Part model, mm, in its own coordinate system. Face numbers are marked on the shaded views. A direction names the side the tool comes from. Coordinates: 2 decimals unless noted, no trailing zeros. Loops run counter-clockwise (first coordinate to the right, second up) from the corner with the lowest first, then second, coordinate; pieces in that order, holes last. Notation, with made-up numbers: M 54.25,-12 L 63.25,-12 A29 cw 63.25,12 Z; hole C 18,30.25 d10. An arc over 180 degrees is marked long. Use a Markdown table: item, result. Add a question column.
1) Tool access for the marked faces 1 and 2: list every direction of +Z, -Z, +X, -X, +Y, -Y with a clear straight run to the whole face (end or side of a thin tool).
2) Band-saw the part on C-C (y = -3). List the corners of the cut face in (x, z).
3) Band-saw the part on D-D (z = 6). List the corners of the cut face in (x, y).
4) Pull direction Z, two halves, no side cores. Call the marked faces 3, 4 and 5: released by +Z, released by -Z, zero draft, split by the parting line, or undercut.
5) Band-saw the part on A-A (x = 0). List the corners of the cut face in (y, z), plus the area to 3 significant figures.
6) Wall check: probe 1 along Y at (x, z) = (0, 4.25); probe 2 along Y at (x, z) = (0, 0.35). Give the ranges that are in metal, low to high. Write a range as from..to.
7) Pin check, flat tips, straight feed: pin 1 Ø3 at (x, y) = (0, 0) entering from +Z; pin 2 Ø1.5 at (y, z) = (2.5, 2) entering from -X; pin 3 Ø3 at (x, z) = (6, 2.5) entering from -Y; pin 4 Ø4.5 at (x, y) = (3.5, -3.5) entering from +Z. Stop position of each tip, or through.
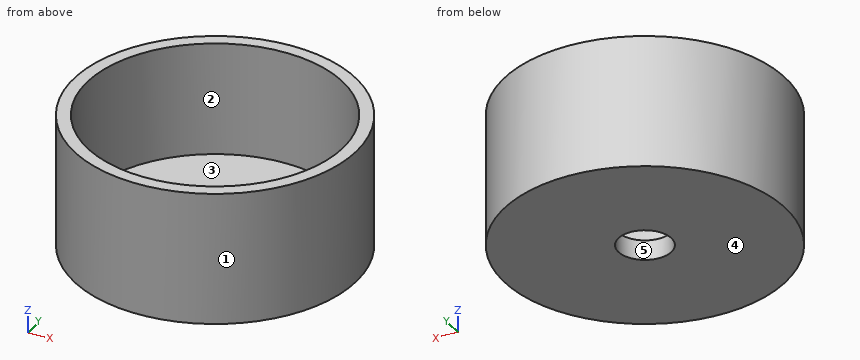
Autodesk Inventor part; units mm, degrees
ref_plane "YZ Plane" through (0, 0, 0) normal (1, 0, 0) x (0, 1, 0)
ref_plane "XZ Plane" through (0, 0, 0) normal (0, 1, 0) x (-1, 0, 0)
ref_plane "XY Plane" through (0, 0, 0) normal (0, 0, 1) x (1, 0, 0)
sketch "Sketch1" plane through (0, 0, 0) normal (0, 0, 1) x (1, 0, 0)
  circle A0 centre (0, 0) radius 8.5
  dimension "d0" = 17
extrude "Extrusion1" add sketch "Sketch1" along normal blind 8
sketch "Sketch2" plane through (0, 0, 8) normal (0, 0, 1) x (1, 0, 0)
  circle A0 centre (0, 0) radius 7.7
  circle A1 centre (0, 0) radius 8.5
  dimension "d3" = 0.8
extrude "Extrusion2" cut sketch "Sketch2" against normal blind 6.8 contours A0
sketch "Sketch3" plane through (0, 0, 0) normal (0, 0, -1) x (-1, 0, 0)
  point P0 (0, 0)
hole "Hole1" at (0, 0, 0) direction (0, 0, 1) diameter 3.2 end through all
properties part number "SpoolSpringBushing"
Entries:
| question | item | result |
|---|---|---|
| 1 | face 1 | +Z, -Z |
| 1 | face 2 | +Z |
| 2 | outline | M -7.95,0 L 7.95,0 L 7.95,8 L 7.09,8 L 7.09,1.2 L -7.09,1.2 L -7.09,8 L -7.95,8 Z |
| 3 | outline | C 0,0 d17; hole C 0,0 d15.4 |
| 4 | face 3 | released by +Z |
| 4 | face 4 | released by -Z |
| 4 | face 5 | zero draft |
| 5 | outline | M -8.5,0 L -1.6,0 L -1.6,1.2 L -7.7,1.2 L -7.7,8 L -8.5,8 Z; M 1.6,0 L 8.5,0 L 8.5,8 L 7.7,8 L 7.7,1.2 L 1.6,1.2 Z |
| 5 | area | 27.4 mm2 |
| 6 | probe 1 | -8.5..-7.7, 7.7..8.5 |
| 6 | probe 2 | -8.5..-1.6, 1.6..8.5 |
| 7 | pin 1 | through |
| 7 | pin 2 | x = -8.32 |
| 7 | pin 3 | y = -7.21 |
| 7 | pin 4 | z = 1.2 |
